The listing builds one solid part. Answer for the finished solid, in the listing's coordinates (mm). Face numbers are marked on the shaded views. A direction names the side the tool comes from. Round coordinates to 2 decimals unless told otherwise and drop trailing zeros. Order: outer loops, then holes, each group sorted by start corner. A loop starts at its lowest first (then second) coordinate and runs counter-clockwise, first axis right, second up. Notation, with made-up numbers: (-24, 50) - (2, 50) arc R29 cw to (2, 79) - close; hole circle Ø8 at (11, 73.5). An arc over 180 degrees is marked (long way). Use CSV: the item, a comma, the result in double quotes. Start each with the question number.
Item 1: Find section D-D, the plane y = 26. Give the vertices of the cut face in (x, z).
Item 2: Find section B-B, the plane z = 3. Give the vertices of the cut face in (x, y), plus the area to 3 significant figures.
Item 3: Flat-ended cylindrical pins translate along their axes: P1, Ø3, axis at x = 13.5, y = 26.5, coming from the +Z side; P2, Ø10, axis at x = 23, y = 20, coming from the +Z side; P3, Ø2, axis at x = 26.5, y = 15, coming from the +Z side. Find the tip coordinate at first contact, or state that the pin passes through.
Item 4: Find section C-C, the plane x = 3. Give the vertices of the cut face in (y, z).
Item 5: For the marked faces 5 and 6, determine the directions among +Z, -Z, +X, -X, +Y, -Y from which every point of the face is accessible in a straight line to the end or side of a thin tool.
Item 6: Straight lines are drawn through the part: line 1 along Y through (x, z) = (8, 3.5); line 2 along X through (y, z) = (39, 5); line 3 along X through (y, z) = (42.6, 3). For each, find the intervals that lie inside material, in ascending order. Write a range as [from, to].
Item 7: Find section A-A, the plane y = 5. Give the vertices of the cut face in (x, z) (1 decimal), plus the area to 3 significant figures.
Item 8: Determine the mould class of the marked faces 1, 2, 3 and 4 for opening direction Z: +Z half, -Z half, draft (parallel to the pull), parting line (faces both ways), or undercut.
```python
from build123d import *

# Parameters (mm, degrees)
BOSS_EXTRUDE1_DEPTH = 46
CUT_EXTRUDE3_START  = -16
CUT_EXTRUDE3_DEPTH  = 25
SKETCH3_R           = 1.5875
CUT_EXTRUDE4_DEPTH  = 65.070116259
SKETCH5_R           = 2.5
CUT_EXTRUDE5_DEPTH  = 10


with BuildPart() as part:
    # Sketch1 → Boss-Extrude1 (new body)
    with BuildSketch(Plane(origin=(0, 0, 0), x_dir=(1, 0, 0), z_dir=(0, 1, 0))):
        Polygon((0, 0), (0, -28), (3.535533906, -31.535533906), (31.535533906, -3.535533906), (28, 0), align=None)
    extrude(amount=BOSS_EXTRUDE1_DEPTH)

    # Sketch2 → Cut-Extrude3 (cut)
    with BuildSketch(Plane.XZ.offset(CUT_EXTRUDE3_START)):
        with BuildLine():
            Line((0, 20), (0, 0))
            Line((0, 0), (20, 0))
            ThreePointArc((20, 0), (14.142135624, 14.142135624), (0, 20))
        make_face()
    extrude(amount=-CUT_EXTRUDE3_DEPTH, mode=Mode.SUBTRACT)

    # Sketch3 → Cut-Extrude4 (cut, through all)
    with BuildSketch(Plane(origin=(0, 46, 0), x_dir=(1, 0, 0), z_dir=(0, 1, 0))):
        with Locations(Location((3, -3, 0), (0, 0, 270))):
            Circle(SKETCH3_R)
    extrude(amount=-CUT_EXTRUDE4_DEPTH, mode=Mode.SUBTRACT)

    # Sketch5 → Cut-Extrude5 (cut)
    with BuildSketch(Plane(origin=(0, 46, 0), x_dir=(1, 0, 0), z_dir=(0, 1, 0))):
        with Locations(Location((25.313708499, -4.100505063, 0), (0, 0, 270))):
            Circle(SKETCH5_R)
        with Locations(Location((4.100505063, -25.313708499, 0), (0, 0, 90))):
            Circle(SKETCH5_R)
    extrude(amount=-CUT_EXTRUDE5_DEPTH, mode=Mode.SUBTRACT)


solid = part.part
```
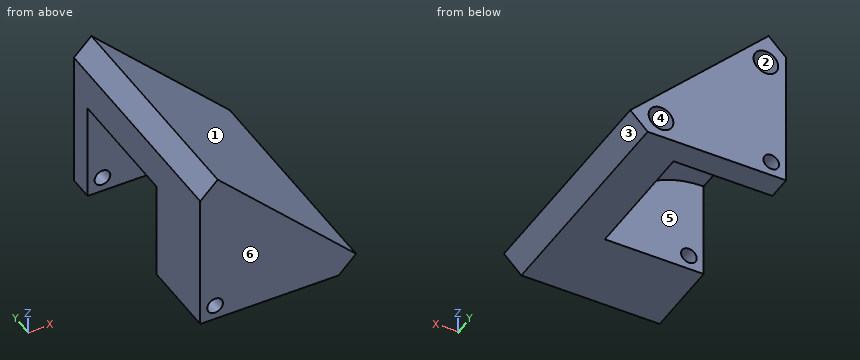
Worked out:
1,outline,"(0, 20) arc R20 cw to (20, 0) - (28, 0) - (31.54, 3.54) - (3.54, 31.54) - (0, 28) - close"
2,outline,"(0, 0) - (1.41, 0) - (1.41, 16) - (0, 16) - close; (0, 41) - (1.41, 41) - (1.41, 46) - (0, 46) - close; (4.59, 0) - (31, 0) - (31, 46) - (27.56, 46) - (27.56, 36) - (23.07, 36) - (23.07, 46) - (4.59, 46) - (4.59, 41) - (19.77, 41) - (19.77, 16) - (4.59, 16) - close"
2,area,"820 mm²"
3,P1,"stops at z = 23.07"
3,P2,"stops at z = 17.07"
3,P3,"stops at z = 9.57"
4,outline,"(0, 0) - (16, 0) - (16, 1.41) - (0, 1.41) - close; (0, 4.59) - (16, 4.59) - (16, 19.77) - (41, 19.77) - (41, 4.59) - (46, 4.59) - (46, 23.07) - (36, 23.07) - (36, 27.56) - (46, 27.56) - (46, 31) - (0, 31) - close; (41, 0) - (46, 0) - (46, 1.41) - (41, 1.41) - close"
5,face 5,"-Z, -X"
5,face 6,"+Z, -Z, +X, -X, -Y"
6,line 1,"y = [0, 16], [41, 46]"
6,line 2,"x = [19.36, 22.98], [27.65, 30.07]"
6,line 3,"x = [0, 1.41], [4.59, 23.07], [27.56, 31]"
7,outline,"(0, 0) - (28, 0) - (31.5, 3.5) - (3.5, 31.5) - (0, 28) - close; hole circle Ø3.2 at (3, 3)"
7,area,"582 mm²"
8,face 1,"+Z half"
8,face 2,"undercut"
8,face 3,"-Z half"
8,face 4,"undercut"
